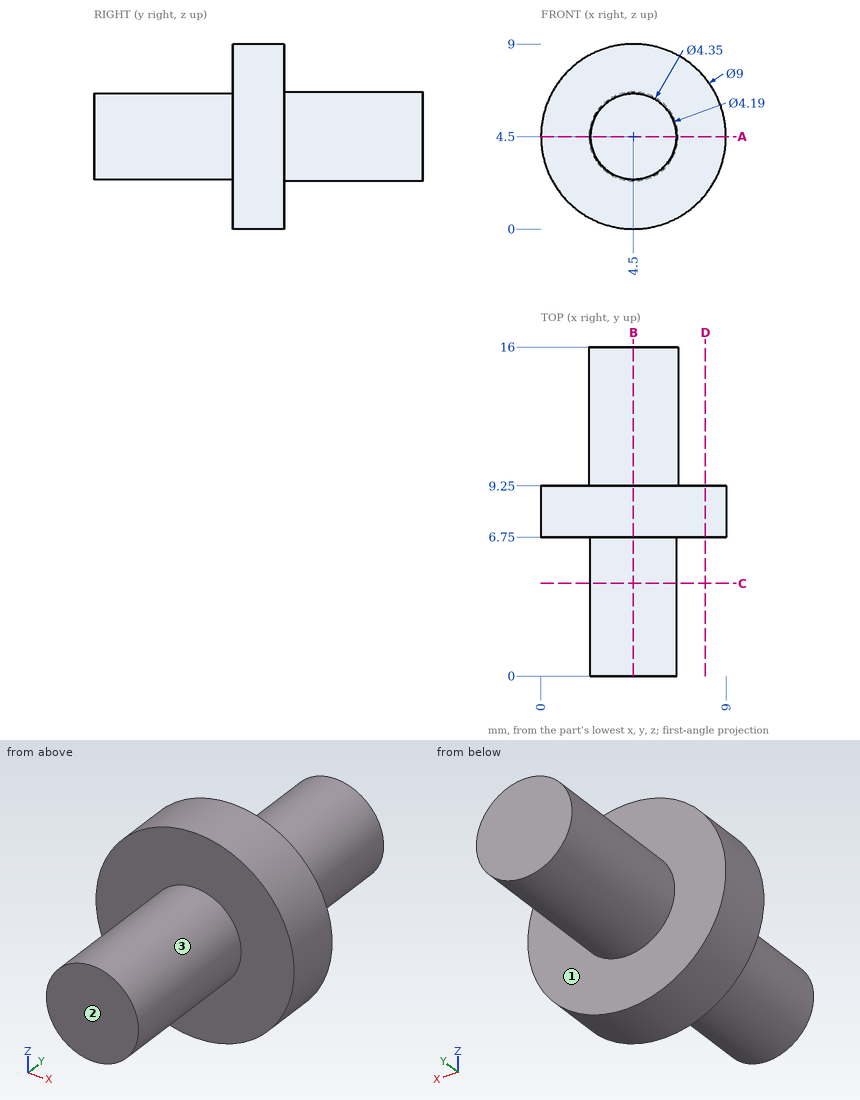
Answer from the drawing. Dimensions are ordinates in mm from the lowest x, y and z of the part. A direction names the side the tool comes from. Round coordinates to 2 decimals unless told otherwise and drop trailing zeros. Write each loop counter-clockwise with the first axis right and the second up, starting at its lowest first coordinate (ties: lowest second). Pieces come first, ordered by that corner, then holes. Notation, with made-up numbers: (12, -36) - (39, -36) arc R8 cw to (39, -25) - close; hole circle Ø6 at (43, 20). An arc over 180 degrees is marked (long way). Use a Markdown table: item, result.
(1) The part is cut by section B-B (x = 4.5). Write down the section's boundary in (y, z) (3 decimals), then the cut area to 3 significant figures.
Reported:
| item | result |
|---|---|
| outline | (0, 2.405) - (6.75, 2.405) - (6.75, 0) - (9.25, 0) - (9.25, 2.325) - (16, 2.325) - (16, 6.675) - (9.25, 6.675) - (9.25, 9) - (6.75, 9) - (6.75, 6.595) - (0, 6.595) - close |
| area | 80.1 mm2 |
(2) Which of the six approach directions +Z, -Z, +X, -X, +Y, -Y give full straight-line access (tool end or side, diameter ignored) to the marked faces 1, 2 and 3?
Reported:
| item | result |
|---|---|
| face 1 | +Y |
| face 2 | +Z, -Z, +X, -X, -Y |
| face 3 | -Y |
(3) Straight lines are drawn through the part: line 1 along Y through (x, z) = (8, 3.25); line 2 along X through (y, z) = (10, 4.5) (3 decimals); line 3 along Z through (x, y) = (7.5, 7.5). For each, find the intervals that lie inside material, in ascending order. Write a range as [from, to].
Reported:
| item | result |
|---|---|
| line 1 | [6.75, 9.25] |
| line 2 | [2.325, 6.675] |
| line 3 | [1.15, 7.85] |
(4) The part is cut by section C-C (y = 4.5). Write down the section's boundary in (x, z) (3 decimals), then the cut area to 3 significant figures.
Reported:
| item | result |
|---|---|
| outline | circle Ø4.19 at (4.5, 4.5) |
| area | 13.8 mm2 |
(5) The part is cut by section D-D (x = 8). Write down the section's boundary in (y, z), then the cut area to 3 significant figures.
Reported:
| item | result |
|---|---|
| outline | (6.75, 1.67) - (9.25, 1.67) - (9.25, 7.33) - (6.75, 7.33) - close |
| area | 14.1 mm2 |
(6) Each of these flat-tipped pins is pushed along its axis until it touches: pin 1 Ø2 at (x, z) = (2.5, 1) entering from +Y; pin 2 Ø2 at (x, y) = (5.5, 13) entering from -Z (3 decimals); pin 3 Ø3 at (y, z) = (10.5, 1.5) entering from +X. Where does it stop, or does it pass through?
Reported:
| item | result |
|---|---|
| pin 1 | y = 9.25 |
| pin 2 | z = 2.325 |
| pin 3 | x = 8.44 |
(7) The part is cut by section A-A (z = 4.5). Write down the section's boundary in (x, y) (3 decimals).
Reported:
| item | result |
|---|---|
| outline | (0, 6.75) - (2.405, 6.75) - (2.405, 0) - (6.595, 0) - (6.595, 6.75) - (9, 6.75) - (9, 9.25) - (6.675, 9.25) - (6.675, 16) - (2.325, 16) - (2.325, 9.25) - (0, 9.25) - close |
